from build123d import *

# Parameters (mm, degrees)
F0_R     = 1.905
F1_DEPTH = 25.4
F2_W     = 30.2913453197
F2_H     = 17.5393885002
F4_DEPTH = 1.6891


with BuildPart() as f1:
    # F0 (on Top) → F1 (new body, symmetric)
    with BuildSketch(Plane.XY):
        with Locations((-29.5697990805, 21.6293018311)):
            Circle(F0_R)
    extrude(amount=F1_DEPTH, both=True)


with BuildPart() as f1_1:
    # F3: moved
    add(f1.part.moved(Location((0, -21.844, 0))))

    # F2 (on Front) → F4 (join)
    with BuildSketch(Plane.XZ):
        with Locations((-13.8722935808, 15.2848851867)):
            Rectangle(F2_W, F2_H)
        with BuildLine():
            Line((-6.5367437352, 12.7834337886), (-3.1749898142, 22.2440018152))
            Line((-3.1749898142, 22.2440018152), (-1.3363293843, 22.2440018152))
            Line((-1.3363293843, 22.2440018152), (-6.6365659302, 7.5314983048))
            Line((-6.6365659302, 7.5314983048), (-8.3271031031, 7.5314983048))
            Line((-8.3271031031, 7.5314983048), (-13.6015790825, 22.2440018152))
            Line((-13.6015790825, 22.2440018152), (-11.788679219, 22.2440018152))
            Line((-11.788679219, 22.2440018152), (-8.4076048732, 12.7254725141))
            add(Edge.make_bspline(
                [(-8.4076048732, 12.7254725141), (-7.8247720574, 11.0832364033), (-7.483444552, 9.5343823459)],
                knots=[0, 0, 0, 1, 1, 1], degree=2))
            add(Edge.make_bspline(
                [(-7.483444552, 9.5343823459), (-7.119576551, 11.1637381734), (-6.5367437352, 12.7834337886)],
                knots=[0, 0, 0, 1, 1, 1], degree=2))
        make_face(mode=Mode.SUBTRACT)
    extrude(amount=-F4_DEPTH)


solid = f1_1.part
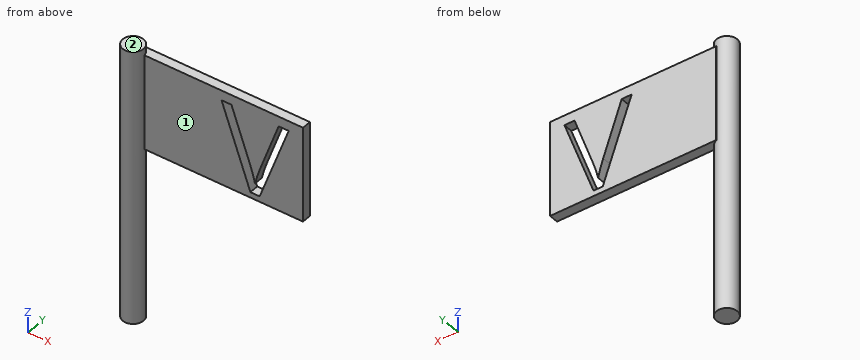
Here's how the part is built. I have some questions about the finished solid (model axes, mm). Face numbers are marked on the shaded views. A direction names the side the tool comes from. Coordinates: 2 decimals unless noted, no trailing zeros. Order: outer loops, then holes, each group sorted by start corner. A loop starts at its lowest first (then second) coordinate and runs counter-clockwise, first axis right, second up. Notation, with made-up numbers: (47, -29.75) - (89, -29.75) arc R25 cw to (89, -2.75) - close; hole circle Ø3 at (41.5, 77). An arc over 180 degrees is marked (long way). Use CSV: the item, a comma, the result in double quotes. Start each with the question number.
1. I'm going to push flat-ended pins straight in: pin 1 (1.4 mm diameter, centred on x = -10.5, y = 1, fed in from +Z); pin 2 (0.5 mm diameter, centred on x = -12.5, y = 1, fed in from -Z); pin 3 (8 mm diameter, centred on x = -10.5, z = 6.5, fed in from -Y). Where does each tip first touch, or does it pass through?
2. Suppose I cut it at D-D on y = -1. List the corners of the cut face in (x, z) for me, then the cut area to 3 significant figures.
3. For the marked faces 1 and 2, which set-ups out of +Z, -Z, +X, -X, +Y, -Y let a thin tool reach every point of the face, with its end or its side?
4. Please list where these lines run through material, in increasing order: line 1 (X direction, y = 1.1, z = 15); line 2 (X direction, y = 0.5, z = 17); line 3 (Z direction, x = -17.5, y = 1.1). Write a range as from..to.
5. Suppose I cut it at C-C on x = -21.5. List the corners of the cut face in (y, z) for me.
6. Suppose I cut it at B-B on z = 18.5. List the corners of the cut face in (x, y) for me (3 decimals).
7. Suppose I cut it at A-A on z = 7. List the corners of the cut face in (x, y) for me (3 decimals).
Output:
1,pin 1,"stops at z = 24.05"
1,pin 2,"stops at z = 6.52"
1,pin 3,"stops at y = 0"
2,outline,"(-31.31, -25.4) - (-27.83, -25.4) - (-27.83, 25.4) - (-31.31, 25.4) - close"
2,area,"176 mm2"
3,face 1,"+Z, -Z, +X, -Y"
3,face 2,"+Z, +X, -X, +Y, -Y"
4,line 1,"x = -30.95..-11, -9.22..-5.75, -3.95..1.27"
4,line 2,"x = -31.34..-11.72, -9.93..-5.04, -3.23..1.27"
4,line 3,"z = 6.52..24.05"
5,outline,"(0, 6.52) - (1.69, 6.52) - (1.69, 24.05) - (0, 24.05) - close"
6,outline,"(-29.018, 1.609) arc R1.905 ccw (long way) to (-27.677, 0) - (-12.259, 0) - (-12.259, 1.689) - (-29.018, 1.689) - close; (-10.459, 0) - (-4.505, 0) - (-4.505, 1.689) - (-10.459, 1.689) - close; (-2.685, 0) - (1.273, 0) - (1.273, 1.689) - (-2.685, 1.689) - close"
7,outline,"(-29.018, 1.609) arc R1.905 ccw (long way) to (-27.677, 0) - (1.273, 0) - (1.273, 1.689) - (-29.018, 1.689) - close"
